from build123d import *


with BuildPart() as part:
    # Sketch1 → Base-Revolve (revolve)
    with BuildSketch(Plane.XY):
        with BuildLine():
            Line((134.323673019, 32.5), (-9.4019e-05, 32.5))
            Line((-9.4019e-05, 32.5), (-131.1, 32.5))
            ThreePointArc((-131.1, 32.5), (-131.382842712, 32.382842712), (-131.5, 32.1))
            Line((-131.5, 32.1), (-131.5, 28.4))
            ThreePointArc((-131.5, 28.4), (-131.617157288, 28.117157288), (-131.9, 28))
            Line((-131.9, 28), (-132.5, 28))
            Line((-132.5, 28), (-132.5, 25.230940108))
            ThreePointArc((-132.5, 25.230940108), (-132.553589838, 25.030940108), (-132.7, 24.884529946))
            Line((-132.7, 24.884529946), (-136.3, 22.806068977))
            ThreePointArc((-136.3, 22.806068977), (-136.446410162, 22.659658816), (-136.5, 22.459658816))
            Line((-136.5, 22.459658816), (-136.5, 5.1))
            Line((-136.5, 5.1), (-116.5, 5.1))
            Line((-116.5, 5.1), (-113.555513627, 0))
            Line((-113.555513627, 0), (136.5, 0))
            Line((136.5, 0), (136.5, 31.071851993))
            ThreePointArc((136.5, 31.071851993), (136.319152044, 31.64542843), (135.842020143, 32.011544614))
            Line((135.842020143, 32.011544614), (134.665693163, 32.439692621))
            ThreePointArc((134.665693163, 32.439692621), (134.497321197, 32.484807753), (134.323673019, 32.5))
        make_face()
    revolve(axis=Axis((-136.5, 0, 0), (1, 0, 0)))


solid = part.part
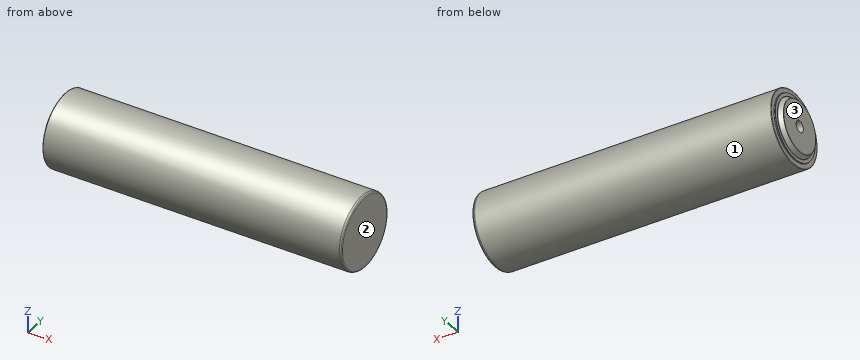
Design review of the part built by this model. Coordinates are the model's own, in mm. Face numbers are marked on the shaded views. Coordinates: 2 decimals unless noted, no trailing zeros. Order: outer loops, then holes, each group sorted by start corner. A loop starts at its lowest first (then second) coordinate and runs counter-clockwise, first axis right, second up. Notation, with made-up numbers: (-9, 9.5) -> (6, 9.5) arc R8 ccw to (6, 20.5) -> close; hole circle Ø5 at (88.25, 88.25). An arc over 180 degrees is marked (long way). One line per item, written item: value.
1) We need section A-A, the plane x = -102. Give the boundary of the cut face in (y, z), then the cut area to 3 significant figures.
Output values:
outline: circle Ø65 at (0, 0)
area: 3,320 mm2
2) Draft analysis for pull direction X (two halves, no side actions). For the marked faces 1, 2 and 3, state which applies: +X half, -X half, draft (parallel to the pull), parting line (faces both ways), or undercut.
Output values:
face 1: draft
face 2: +X half
face 3: -X half
3) Clearance check with flat-ended pins moving along their axes: P1, Ø8, axis at x = 68, z = 21.5, coming from the +Y side; P2, Ø8, axis at x = 95, y = 20, coming from the +Z side; P3, Ø12, axis at x = 107.5, y = -18.5, coming from the -Z side; P4, Ø10, axis at x = 11, z = -0.5, coming from the -Y side. State where each tip first meets the part, or that it passes through.
Output values:
P1: stops at y = 27.39
P2: stops at z = 28.29
P3: stops at z = -30
P4: stops at y = -32.5
4) To check wall thickness, follow probe 1 along Z at (x, y) = (-122, 0); probe 2 along Y at (x, z) = (60, 16.5); probe 3 along X at (y, z) = (-29, -2). State the ranges of each line that lie inside material, in increasing order. Write a range as [from, to].
Output values:
probe 1: z = [-32.5, -5.1], [5.1, 32.5]
probe 2: y = [-28, 28]
probe 3: x = [-131.5, 136.5]
